```python
from build123d import *

# Parameters (mm, degrees)
F0_W     = 40
F0_H     = 40
F0_W_2   = 36
F0_H_2   = 36
F1_DEPTH = 200
F2_W     = 10
F2_H     = 30
F3_DEPTH = 20.001
F4_R     = 5
F5_DEPTH = 20.001


# Not quite as in the source:
# - a pattern or mirror of a feature is missing from the dataset's text; its kind, count and spacing are read off the source's solid


with BuildPart() as f1:
    # F0 (on Front) → F1 (new body, symmetric)
    with BuildSketch(Plane.XZ):
        Rectangle(F0_W, F0_H)
        Rectangle(F0_W_2, F0_H_2, mode=Mode.SUBTRACT)
    extrude(amount=F1_DEPTH, both=True)

    # F2 (on Right) → F3 (cut, through all)
    with BuildSketch(Plane.YZ):
        with Locations((-190, 15)):
            Rectangle(F2_W, F2_H)
    f3 = extrude(amount=-F3_DEPTH, mode=Mode.SUBTRACT)

    # F3_copies: F3 across plane
    add(f3.mirror(Plane.ZX), mode=Mode.SUBTRACT)

    # F4 (on Top) → F5 (cut, through all)
    with BuildSketch(Plane.XY):
        with Locations((-10, 170)):
            Circle(F4_R)
    f5 = extrude(amount=F5_DEPTH, mode=Mode.SUBTRACT)

    # F5_copies: F5 across plane
    add(f5.mirror(Plane(origin=(0, 0, 0), x_dir=(0, 0, -1), z_dir=(0, -1, 0))), mode=Mode.SUBTRACT)


solid = f1.part
```
Could you check a few things on this model? Use its own coordinates, in mm. A direction names the side the tool comes from. Coordinates: 2 decimals unless noted, no trailing zeros. Write each loop counter-clockwise with the first axis right and the second up, starting at its lowest first coordinate (ties: lowest second). Pieces come first, ordered by that corner, then holes. Notation, with made-up numbers: (-25, 25.5) -> (24, 25.5) arc R7 ccw to (24, 35.5) -> close; hole circle Ø9 at (30, 21). An arc over 180 degrees is marked (long way). Write item = value, one per line. Start each with the question number.
(1) I want a section at C-C (z = 6.5). Please give me the cut outline in (x, y), plus the area to 3 significant figures.
(2) I want a section at B-B (x = 13). Please give me the cut outline in (y, z), plus the area to 3 significant figures.
(3) I need wall thicknesses on line 1 (Y direction, x = -10, z = 19.25); line 2 (X direction, y = -40.5, z = -14). Which ranges of each line are inside material? Lowest first, please. Write a range as [from, to].
(4) I want a section at D-D (y = -170). Please give me the cut outline in (x, z), plus the area to 3 significant figures.
(5) Will these pins go through, and if not, where does the flat tip stop? pin 1 (1.6 mm diameter, centred on y = 192.5, z = 19, fed in from -X); pin 2 (1.6 mm diameter, centred on x = -18.5, y = 192, fed in from +Z); pin 3 (9 mm diameter, centred on x = -10, y = -170, fed in from +Z).
(6) We'd pull the mould along Z, two halves only. Please class faces 1 (the face through (0, -3, 20)), 2 (the face through (-19, -185, 14)), 3 (the face through (0, -3, 18)), 4 (the face through (0, -3, -18)): released by +Z, released by -Z, zero draft, split by the parting line, or undercut.
(7) Which directions (+Z, -Z, +X, -X, +Y, -Y) give clear straight access to the entire face, cutting with the end or side of a thin tool? Please do faces 5 (the face through (-10.651, -174.957, 18.986)), 6 (the face through (-18, -3, 0)), 7 (the face through (-19, 185, 14)), 8 (the face through (-20, -3, 0)).
(8) I want a section at A-A (x = -10). Please give me the cut outline in (y, z), plus the area to 3 significant figures.
Result set:
q1.outline = (-20, -200) -> (-18, -200) -> (-18, -195) -> (-20, -195) -> close; (-20, -185) -> (-18, -185) -> (-18, 185) -> (-20, 185) -> close; (-20, 195) -> (-18, 195) -> (-18, 200) -> (-20, 200) -> close; (18, -200) -> (20, -200) -> (20, 200) -> (18, 200) -> close
q1.area = 1,560 mm2
q2.outline = (-200, -20) -> (200, -20) -> (200, -18) -> (-200, -18) -> close; (-200, 18) -> (200, 18) -> (200, 20) -> (-200, 20) -> close
q2.area = 1,600 mm2
q3.line_1 = [-200, -195], [-185, -175], [-165, 165], [175, 185], [195, 200]
q3.line_2 = [-20, -18], [18, 20]
q4.outline = (-20, -20) -> (20, -20) -> (20, 20) -> (-5, 20) -> (-5, 18) -> (18, 18) -> (18, -18) -> (-18, -18) -> (-18, 18) -> (-15, 18) -> (-15, 20) -> (-20, 20) -> close
q4.area = 284 mm2
q5.pin_1 = 0
q5.pin_2 = 0
q5.pin_3 = -18
q6.face_1 = released by +Z
q6.face_2 = zero draft
q6.face_3 = undercut
q6.face_4 = undercut
q7.face_5 = +Z
q7.face_6 = +Y, -Y
q7.face_7 = +Z, -X
q7.face_8 = +Z, -Z, -X, +Y, -Y
q8.outline = (-200, -20) -> (200, -20) -> (200, -18) -> (-200, -18) -> close; (-200, 18) -> (-195, 18) -> (-195, 20) -> (-200, 20) -> close; (-185, 18) -> (-175, 18) -> (-175, 20) -> (-185, 20) -> close; (-165, 18) -> (165, 18) -> (165, 20) -> (-165, 20) -> close; (175, 18) -> (185, 18) -> (185, 20) -> (175, 20) -> close; (195, 18) -> (200, 18) -> (200, 20) -> (195, 20) -> close
q8.area = 1,520 mm2
